Check sheet for the modelled part. Datum: model origin and axes. Units: mm. A direction names the side the tool comes from. Coordinates: 2 decimals unless noted, no trailing zeros. Loops run counter-clockwise (first coordinate to the right, second up) from the corner with the lowest first, then second, coordinate; pieces in that order, holes last. Notation, with made-up numbers: (34.25, 38.5) - (83.25, 38.5) arc R21 ccw to (83.25, 43.5) - close; hole circle Ø6 at (20, -29.75). An arc over 180 degrees is marked (long way). Answer as a JSON object with one key per item and string values. Group by question number.
from build123d import *

# Parameters (mm, degrees)
F0_R      = 8
F1_DEPTH  = 3.8
F2_R      = 6.15
F3_DEPTH  = 5.9
F4_R      = 8
F5_DEPTH  = 7
F6_R      = 11.15
F7_DEPTH  = 25.7
F8_R      = 2.5
F9_DEPTH  = 3
F10_W     = 20
F10_H     = 16
F10_R     = 2.5
F11_DEPTH = 12
F13_DEPTH = 5
F14_SIZE  = 3


with BuildPart() as f1:
    # F0 (on Top) → F1 (new body)
    with BuildSketch(Plane.XY):
        Circle(F0_R)
    extrude(amount=-F1_DEPTH)

    # F2 (on face) → F3 (join)
    with BuildSketch(Plane(origin=(0, 0, -3.8), x_dir=(1, 0, 0), z_dir=(0, 0, -1))):
        Circle(F2_R)
    extrude(amount=F3_DEPTH)

    # F4 (on face) → F5 (join)
    with BuildSketch(Plane(origin=(0, 0, -9.7), x_dir=(1, 0, 0), z_dir=(0, 0, -1))):
        Circle(F4_R)
    extrude(amount=F5_DEPTH)

    # F6 (on face) → F7 (join)
    with BuildSketch(Plane(origin=(0, 0, -16.7), x_dir=(1, 0, 0), z_dir=(0, 0, -1))):
        Circle(F6_R)
    extrude(amount=F7_DEPTH)

    # F8 (on face) → F9 (join)
    with BuildSketch(Plane(origin=(0, 0, -42.4), x_dir=(1, 0, 0), z_dir=(0, 0, -1))):
        Circle(F8_R)
    extrude(amount=F9_DEPTH)

    # F10 (on face) → F11 (join)
    with BuildSketch(Plane(origin=(0, 0, -45.4), x_dir=(1, 0, 0), z_dir=(0, 0, -1))):
        with Locations((6, 0)):
            Rectangle(F10_W, F10_H)
        Circle(F10_R, mode=Mode.SUBTRACT)
        Circle(F10_R)
    extrude(amount=F11_DEPTH)

    # F12 (on face) → F13 (join)
    with BuildSketch(Plane(origin=(0, 0, -57.4), x_dir=(1, 0, 0), z_dir=(0, 0, -1))):
        Polygon((0, -4.041452), (3.5, -2.020726), (3.5, 2.020726), (0, 4.041452), (-3.5, 2.020726), (-3.5, -2.020726), align=None)
    extrude(amount=F13_DEPTH)

    # F14
    f14_edges = [f1.edges().sort_by_distance(p)[0] for p in [
        (3.5, 0, -62.4),
        (1.75, -3.031089, -62.4),
        (-1.75, -3.031089, -62.4),
        (-3.5, 0, -62.4),
        (1.75, 3.031089, -62.4),
        (-1.75, 3.031089, -62.4),
    ]]
    chamfer(f14_edges, length=F14_SIZE)


solid = f1.part
1. Sectioned sample at C-C on z = -38.5. Record the cut outline in (x, y), plus the area to 3 significant figures.
2. Material ranges on line 1 (Z direction, x = 3.75, y = -4); line 2 (X direction, y = 0.5, z = -42); line 3 (Z direction, x = -7.25, y = -3.5), recorded low to high.
3. Sectioned sample at B-B on y = 7. Record the cut outline in (x, z).
4. Access from +Z, -Z, +X, -X, +Y, -Y to the whole of each face (thin tool, end or side, straight path). Record for faces 5 (the face through (-1.726, -3.045, -58.386)), 6 (the face through (-4, 0, -51)), 7 (the face through (10.635, -3.349, -29.37)), 8 (the face through (6, -8, -51)), 9 (the face through (-2, -6, -3.8)).
5. Release check for a two-part mould opening along Z. For faces 1 (the face through (-2, 6, -9.7)), 2 (the face through (-1.132, -2.017, -60.588)), 3 (the face through (6, 0, -45.4)), 4 (the face through (1.726, 3.045, -58.386)) record: released by +Z, released by -Z, zero draft, split by the parting line, or undercut.
6. Sectioned sample at D-D on y = -9. Record the cut outline in (x, z), plus the area to 3 significant figures.
7. Gauge pin test, flat ends, axial feed: pin 1 (1.5 mm diameter, centred on x = 11, y = -2.5, fed in from -Z); pin 2 (2 mm diameter, centred on x = 9.5, z = -56, fed in from +Y); pin 3 (10 mm diameter, centred on x = 7, y = 5.5, fed in from -Z). Record the tip position at first contact, or that the pin passes through.
Answers follow:
{
 "1": {"outline": "circle Ø22.3 at (0, 0)", "area": "391 mm^2"},
 "2": {"line 1": "z = -57.4 to -45.4, -42.4 to 0", "line 2": "x = -11.14 to 11.14", "line 3": "z = -42.4 to -16.7"},
 "3": {"outline": "(-8.68, -42.4) - (8.68, -42.4) - (8.68, -16.7) - (3.87, -16.7) - (3.87, -9.7) - (-3.87, -9.7) - (-3.87, -16.7) - (-8.68, -16.7) - close; (-4, -57.4) - (16, -57.4) - (16, -45.4) - (-4, -45.4) - close; (-3.87, -3.8) - (3.87, -3.8) - (3.87, 0) - (-3.87, 0) - close"},
 "4": {"face 5": "-Z, -X, -Y", "face 6": "-Z, -X, +Y, -Y", "face 7": "+Z", "face 8": "-Z, +X, -X, -Y", "face 9": "none"},
 "5": {"face 1": "undercut", "face 2": "released by -Z", "face 3": "undercut", "face 4": "zero draft"},
 "6": {"outline": "(-6.58, -42.4) - (6.58, -42.4) - (6.58, -16.7) - (-6.58, -16.7) - close", "area": "338 mm^2"},
 "7": {"pin 1": "stops at z = -57.4", "pin 2": "stops at y = 8", "pin 3": "stops at z = -59.46"}
}
